Model file for the job. Use its own axes, mm. Give positions to 0.01 mm unless a question says otherwise; leave off trailing zeros. Order: outer loops, then holes, each group sorted by start corner. A loop starts at its lowest first (then second) coordinate and runs counter-clockwise, first axis right, second up. Notation, with made-up numbers: (55, 2.25) -> (83, 2.25) arc R29 cw to (83, 36.25) -> close; hole circle Ø3 at (23, -2). An arc over 180 degrees is marked (long way). Use CSV: the item, a comma, the result in double quotes. Start each with the question number.
1. Cut at C-C on y = 16. List the corners of the cut face in (x, z), then the cut area to 3 significant figures.
2. Wall check: line 1 (X direction, y = 2, z = 1); line 2 (Y direction, x = 4, z = -13). Give the ranges that are in metal, low to high. Write a range as from..to.
3. Cut at A-A on x = 0. List the corners of the cut face in (y, z), then the cut area to 3 significant figures.
4. Cut at B-B on z = 0. List the corners of the cut face in (x, y), then the cut area to 3 significant figures.
5. Drop flat-ended pins along their axis: pin 1 (8 mm diameter, centred on x = -15, z = 17, fed in from +Y); pin 2 (4 mm diameter, centred on x = -17, z = 15, fed in from -Y); pin 3 (1 mm diameter, centred on x = 11.5, y = 169, fed in from +Z); pin 4 (3 mm diameter, centred on x = -1, y = 0, fed in from -Z). Give the stop position or say it passes through.
6. Cut at D-D on z = 15.5. List the corners of the cut face in (x, y), then the cut area to 3 significant figures.
```python
from build123d import *

# Parameters (mm, degrees)
SKETCH1_R            = 24.5
BOSS_EXTRUDE8_DEPTH  = 210
SKETCH1_9_R          = 3.95
BOSS_EXTRUDE9_DEPTH  = 15
BOSS_EXTRUDE10_START = -15
SKETCH1_10_R         = 2.95
BOSS_EXTRUDE10_DEPTH = 16
BOSS_EXTRUDE11_START = 225
SKETCH1_11_R         = 3.95
BOSS_EXTRUDE11_DEPTH = 15
BOSS_EXTRUDE12_START = 24
SKETCH2_R            = 2.95
BOSS_EXTRUDE12_DEPTH = 24


with BuildPart() as part:
    # Sketch1 → Boss-Extrude8 (new body)
    with BuildSketch(Plane(origin=(0, 0, 0), x_dir=(1, 0, 0), z_dir=(0, 1, 0))):
        with Locations(Location((0, 0, 0), (0, 0, 270))):
            Circle(SKETCH1_R)
    extrude(amount=BOSS_EXTRUDE8_DEPTH)

    # Sketch1<9> → Boss-Extrude9 (add)
    with BuildSketch(Plane(origin=(0, 0, 0), x_dir=(1, 0, 0), z_dir=(0, 1, 0))):
        with Locations(Location((0, 0, 0), (0, 0, 270))):
            Circle(SKETCH1_9_R)
    extrude(amount=-BOSS_EXTRUDE9_DEPTH)

    # Sketch1<10> → Boss-Extrude10 (add)
    with BuildSketch(Plane(origin=(0, 0, 0), x_dir=(1, 0, 0), z_dir=(0, 1, 0)).offset(BOSS_EXTRUDE10_START)):
        with Locations(Location((0, 0, 0), (0, 0, 270))):
            Circle(SKETCH1_10_R)
    extrude(amount=-BOSS_EXTRUDE10_DEPTH)

    # Sketch1<11> → Boss-Extrude11 (add)
    with BuildSketch(Plane(origin=(0, 0, 0), x_dir=(1, 0, 0), z_dir=(0, 1, 0)).offset(BOSS_EXTRUDE11_START)):
        with Locations(Location((0, 0, 0), (0, 0, 270))):
            Circle(SKETCH1_11_R)
    extrude(amount=-BOSS_EXTRUDE11_DEPTH)

    # Sketch2 → Boss-Extrude12 (add)
    with BuildSketch(Plane(origin=(0, 225, 0), x_dir=(1, 0, 0), z_dir=(0, 1, 0)).offset(BOSS_EXTRUDE12_START)):
        with Locations(Location((0, 0, 0), (0, 0, 270))):
            Circle(SKETCH2_R)
    extrude(amount=-BOSS_EXTRUDE12_DEPTH)


solid = part.part
```
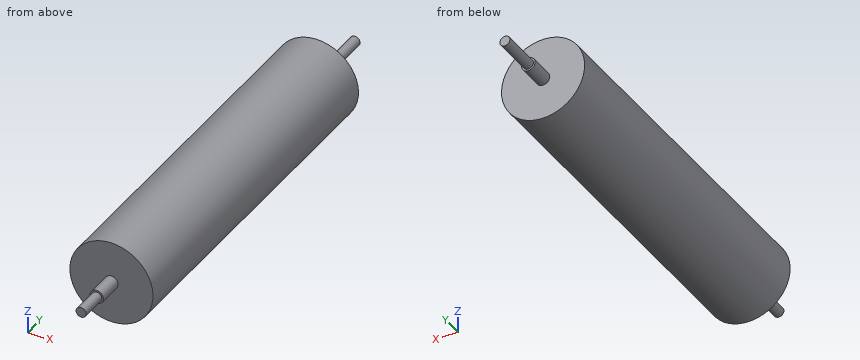
Verdict:
1,outline,"circle Ø49 at (0, 0)"
1,area,"1,890 mm^2"
2,line 1,"-24.48..24.48"
2,line 2,"0..210"
3,outline,"(-31, -2.95) -> (-15, -2.95) -> (-15, -3.95) -> (0, -3.95) -> (0, -24.5) -> (210, -24.5) -> (210, -3.95) -> (225, -3.95) -> (225, -2.95) -> (249, -2.95) -> (249, 2.95) -> (225, 2.95) -> (225, 3.95) -> (210, 3.95) -> (210, 24.5) -> (0, 24.5) -> (0, 3.95) -> (-15, 3.95) -> (-15, 2.95) -> (-31, 2.95) -> close"
3,area,"10,800 mm^2"
4,outline,"(-24.5, 0) -> (-3.95, 0) -> (-3.95, -15) -> (-2.95, -15) -> (-2.95, -31) -> (2.95, -31) -> (2.95, -15) -> (3.95, -15) -> (3.95, 0) -> (24.5, 0) -> (24.5, 210) -> (3.95, 210) -> (3.95, 225) -> (2.95, 225) -> (2.95, 249) -> (-2.95, 249) -> (-2.95, 225) -> (-3.95, 225) -> (-3.95, 210) -> (-24.5, 210) -> close"
4,area,"10,800 mm^2"
5,pin 1,"y = 210"
5,pin 2,"y = 0"
5,pin 3,"z = 21.89"
5,pin 4,"z = -24.5"
6,outline,"(-18.97, 0) -> (18.97, 0) -> (18.97, 210) -> (-18.97, 210) -> close"
6,area,"7,970 mm^2"
